Here's how the part is built. I have some questions about the finished solid (model axes, mm). A direction names the side the tool comes from. Coordinates: 2 decimals unless noted, no trailing zeros. Loops run counter-clockwise (first coordinate to the right, second up) from the corner with the lowest first, then second, coordinate; pieces in that order, holes last. Notation, with made-up numbers: (-32.75, 36) - (14.25, 36) arc R22 cw to (14.25, 73) - close; hole circle Ø6 at (-9, 4). An arc over 180 degrees is marked (long way). Use a Markdown table: item, result.
```python
from build123d import *

# Parameters (mm, degrees)
BOSS_EXTRUDE1_DEPTH = 180
SKETCH2_R           = 5
CUT_EXTRUDE1_DEPTH  = 194.390796058
FILLET1_R           = 2


with BuildPart() as part:
    # Sketch1 → Boss-Extrude1 (new body)
    with BuildSketch(Plane.XY):
        Polygon((0, 0), (0, 50), (50, 50), (50, 0), (48.07222, 0), (48.07222, 48.07222), (1.92778, 48.07222), (1.92778, 0), align=None)
    extrude(amount=BOSS_EXTRUDE1_DEPTH)

    # Sketch2 → Cut-Extrude1 (cut, through all)
    with BuildSketch(Plane.ZY):
        with Locations((10, 25)):
            Circle(SKETCH2_R)
        with Locations((170, 25)):
            Circle(SKETCH2_R)
    extrude(amount=-CUT_EXTRUDE1_DEPTH, mode=Mode.SUBTRACT)

    # Fillet1
    fillet1_edges = [part.edges().sort_by_distance(p)[0] for p in [
        (0, 50, 90),
        (50, 50, 90),
        (48.07222, 48.07222, 90),
        (1.92778, 48.07222, 90),
    ]]
    fillet(fillet1_edges, radius=FILLET1_R)


solid = part.part
```
Q1. I want a section at C-C, the plane y = 25. Write out the boundary of the cut face in (x, z).
Check values:
| item | result |
|---|---|
| outline | (0, 0) - (1.93, 0) - (1.93, 5) - (0, 5) - close; (0, 15) - (1.93, 15) - (1.93, 165) - (0, 165) - close; (0, 175) - (1.93, 175) - (1.93, 180) - (0, 180) - close; (48.07, 0) - (50, 0) - (50, 5) - (48.07, 5) - close; (48.07, 15) - (50, 15) - (50, 165) - (48.07, 165) - close; (48.07, 175) - (50, 175) - (50, 180) - (48.07, 180) - close |
Q2. I want a section at D-D, the plane z = 97. Write out the boundary of the cut face in (x, y).
Check values:
| item | result |
|---|---|
| outline | (0, 0) - (1.93, 0) - (1.93, 46.07) arc R2 cw to (3.93, 48.07) - (46.07, 48.07) arc R2 cw to (48.07, 46.07) - (48.07, 0) - (50, 0) - (50, 48) arc R2 ccw to (48, 50) - (2, 50) arc R2 ccw to (0, 48) - close |
Q3. Please list where these lines run through material, in increasing order: L1, parallel to X at y = 12.5, z = 100; L2, parallel to Y at x = 49, z = 10; L3, parallel to Y at x = 29, z = 17. Write a range as from..to.
Check values:
| item | result |
|---|---|
| L1 | 0..1.93, 48.07..50 |
| L2 | 0..20, 30..49.73 |
| L3 | 48.07..50 |
Q4. I want a section at B-B, the plane y = 5.5. Write out the boundary of the cut face in (x, z), then the cut area to 3 significant figures.
Check values:
| item | result |
|---|---|
| outline | (0, 0) - (1.93, 0) - (1.93, 180) - (0, 180) - close; (48.07, 0) - (50, 0) - (50, 180) - (48.07, 180) - close |
| area | 694 mm^2 |
Q5. If we mould it in two halves opening along X, with no side actions, what happens to faces 3 (the face through (1.928, 23, 89)), 4 (the face through (0, 24, 89)), 5 (the face through (25, 50, 89))? For each: pulls with the +X half, pulls with the -X half, needs draft (parallel to the pull), parting line crosses it, or undercut.
Check values:
| item | result |
|---|---|
| face 3 | undercut |
| face 4 | pulls with the -X half |
| face 5 | needs draft |
Q6. I want a section at A-A, the plane z = 170. Write out the boundary of the cut face in (x, y), then the cut area to 3 significant figures.
Check values:
| item | result |
|---|---|
| outline | (0, 0) - (1.93, 0) - (1.93, 20) - (0, 20) - close; (0, 30) - (1.93, 30) - (1.93, 46.07) arc R2 cw to (3.93, 48.07) - (46.07, 48.07) arc R2 cw to (48.07, 46.07) - (48.07, 30) - (50, 30) - (50, 48) arc R2 ccw to (48, 50) - (2, 50) arc R2 ccw to (0, 48) - close; (48.07, 0) - (50, 0) - (50, 20) - (48.07, 20) - close |
| area | 243 mm^2 |
Q7. Which directions (+Z, -Z, +X, -X, +Y, -Y) give clear straight access to the entire face, cutting with the end or side of a thin tool? Please do faces 1 (the face through (49.023, 20.564, 12.307)), 2 (the face through (25, 48.072, 89)).
Check values:
| item | result |
|---|---|
| face 1 | +X, -X |
| face 2 | +Z, -Z, -Y |
Q8. Will this pin go through, and if not, where does the flat tip stop? P1, Ø2, axis at x = 6.5, z = 94, coming from the -Y side.
Check values:
| item | result |
|---|---|
| P1 | y = 48.07 |
